from build123d import *

# Parameters (mm, degrees)
SKETCH1_R           = 5
SKETCH1_R_2         = 1.5
EXTRUDE1_DEPTH      = 1.5
EXTRUDE2_DEPTH      = 8.228416147
EXTRUDE2_DEPTH_BACK = 8.228416147
SKETCH2_R           = 0.8
SKETCH3_R           = 0.8
EXTRUDE3_DEPTH      = 8.228416147
EXTRUDE4_DEPTH      = 8.228416306
EXTRUDE4_DEPTH_BACK = 8.228416306
SKETCH4_W           = 4.205463009
SKETCH4_H           = 0.572765835
SKETCH4_W_2         = 4.092184544


with BuildPart() as part:
    # Sketch1 → Extrude1 (new, symmetric)
    with BuildSketch(Plane.XY):
        Circle(SKETCH1_R)
        Circle(SKETCH1_R_2, mode=Mode.SUBTRACT)
    extrude(amount=EXTRUDE1_DEPTH, both=True)

    # Sketch2 → Extrude2 (cut, two sides: drawn at the far end of the back side and taken through both)
    with BuildSketch(Plane.XY.offset(-EXTRUDE2_DEPTH_BACK)):
        with Locations((-2.451342218, 2.056920351)):
            Circle(SKETCH2_R)
        with Locations((2.451342218, -2.056920351)):
            Circle(SKETCH2_R)
    extrude(amount=EXTRUDE2_DEPTH + EXTRUDE2_DEPTH_BACK, mode=Mode.SUBTRACT)

    # Sketch3 → Extrude3 (cut, through all)
    with BuildSketch(Plane(origin=(0, 0, 0), x_dir=(1, 0, 0), z_dir=(0, 1, 0))):
        with Locations(Location((0, 0, 0), (0, 0, 270))):
            Circle(SKETCH3_R)
    extrude(amount=-EXTRUDE3_DEPTH, mode=Mode.SUBTRACT)

    # Sketch4 → Extrude4 (cut, two sides: drawn at the far end of the back side and taken through both)
    with BuildSketch(Plane.XY.offset(-EXTRUDE4_DEPTH_BACK)):
        with Locations((-2.102731505, -5.186382918)):
            Rectangle(SKETCH4_W, SKETCH4_H)
        with Locations((2.046092272, -5.186382918)):
            Rectangle(SKETCH4_W_2, SKETCH4_H)
    extrude(amount=EXTRUDE4_DEPTH + EXTRUDE4_DEPTH_BACK, mode=Mode.SUBTRACT)


solid = part.part
For this review, take the finished solid that the model builds, in its own axes (mm). Round coordinates to 2 decimals unless told otherwise and drop trailing zeros. Write each loop counter-clockwise with the first axis right and the second up, starting at its lowest first coordinate (ties: lowest second). Pieces come first, ordered by that corner, then holes. Notation, with made-up numbers: (16.25, 8.5) - (74.25, 8.5) arc R17 ccw to (74.25, 33.5) - close; hole circle Ø10 at (37, 82.25). An arc over 180 degrees is marked (long way). Write item = value, one per line. Start each with the question number.
1. Consider section D-D on y = -4. State the section outline as (x, z) points.
2. Draft analysis for pull direction Z (two halves, no side actions). For faces 1 (the face through (0, -3.1, -0.8)), 2 (the face through (0, -4.9, -1)), 3 (the face through (-1.2, 1.2, 1.5)), 4 (the face through (-1.2, 1.2, -1.5)), state which applies: released by +Z, released by -Z, zero draft, split by the parting line, or undercut.
3. Wall thickness on L1, parallel to X at y = -2, z = -0.3; L2, parallel to X at y = -2, z = -0.55; L3, parallel to Z at x = 0, y = -2.9: over which ranges is each line inside the solid? List them lowest first.
4. Consider section B-B on x = 0. State the section outline as (y, z) points, plus the area to 3 significant figures.
5. Consider section C-C on z = 0.45. State the section outline as (x, y) points.
6. Consider section A-A on y = 0. State the section outline as (x, z) points.
Evaluation:
q1.outline = (-3, -1.5) - (3, -1.5) - (3, 1.5) - (-3, 1.5) - close; hole circle Ø1.6 at (0, 0)
q2.face_1 = undercut
q2.face_2 = zero draft
q2.face_3 = released by +Z
q2.face_4 = released by -Z
q3.L1 = -4.58 to -0.74, 0.74 to 1.65, 3.25 to 4.58
q3.L2 = -4.58 to -0.58, 0.58 to 1.65, 3.25 to 4.58
q3.L3 = -1.5 to -0.8, 0.8 to 1.5
q4.outline = (-4.9, -1.5) - (-1.5, -1.5) - (-1.5, -0.8) - (-4.9, -0.8) - close; (-4.9, 0.8) - (-1.5, 0.8) - (-1.5, 1.5) - (-4.9, 1.5) - close; (1.5, -1.5) - (5, -1.5) - (5, 1.5) - (1.5, 1.5) - close
q4.area = 15.3 mm2
q5.outline = (-0.99, -4.9) - (-0.66, -4.9) - (-0.66, -1.35) arc R1.5 cw (long way) to (0.66, -1.35) - (0.66, -4.9) - (0.99, -4.9) arc R5 ccw (long way) to start; hole circle Ø1.6 at (-2.45, 2.06); hole circle Ø1.6 at (2.45, -2.06)
q6.outline = (-5, -1.5) - (-1.5, -1.5) - (-1.5, 1.5) - (-5, 1.5) - close; (1.5, -1.5) - (5, -1.5) - (5, 1.5) - (1.5, 1.5) - close
